Here's how the part is built. I have some questions about the finished solid (model axes, mm). A direction names the side the tool comes from. Coordinates: 2 decimals unless noted, no trailing zeros. Loops run counter-clockwise (first coordinate to the right, second up) from the corner with the lowest first, then second, coordinate; pieces in that order, holes last. Notation, with made-up numbers: M 45,88 L 69,88 A31 ccw 69,124 Z; hole C -24.5,-20 d11. An arc over 180 degrees is marked long. Use one line per item in the form item = value. Start each with the question number.
(1) On a 3-axis mill with a long thin cutter (end or side, diameter ignored), from which of +Z, -Z, +X, -X, +Y, -Y can I reach the whole of each face in a straight line? I mean faces 4 (the flat face through (-14.2, 4, 3)), 5 (the flat face through (-17, 0, 3)), 6 (the flat face through (0, 10, 0)), 7 (the flat face through (-11.5, -14, 0)). Say none if no direction works.
(2) Imagine slicing it at C-C, the plane y = -11.5. Please give me the cut outline in (x, z).
(3) Thinking about a two-plate mould opening in Y: for faces 1 (the flat face through (18.534, 13.728, 0.01)), 2 (the flat face through (-19, 1, 0)), 3 (the cylindrical face through (-13.706, -14.519, -0.01)), which applies, +Y half, -Y half, draft (parallel to the pull), parting line (faces both ways), or undercut?
(4) Imagine slicing it at A-A, the plane x = 14. Please give me the cut outline in (y, z).
(5) Imagine slicing it at B-B, the plane z = 2.7. Please give me the cut outline in (x, y).
(6) Will these pins go through, and if not, where does the flat tip stop? P1, Ø3.5, axis at x = 14.77, y = -15, coming from the +Z side; P2, Ø0.8, axis at y = -13.5, z = 0, coming from the -X side; P3, Ø0.8, axis at y = -13.5, z = 0, coming from the +X side.
(7) Imagine slicing it at D-D, the plane y = 15. Please give me the cut outline in (x, z) (3 decimals), and give its area (3 significant figures).
(8) Please list where these lines run through material, in increasing order: L1, parallel to Y at x = -14.5, z = 1.55; L2, parallel to Z at x = -7.5, y = 6.5; L3, parallel to Y at x = -4.5, z = -0.1.
```python
from build123d import *

# Parameters (mm, degrees)
F0_R     = 1.6
F1_DEPTH = 0.75
F2_W     = 5
F2_H     = 8
F3_DEPTH = 4
F4_W     = 7.2
F4_H     = 3.6
F5_DEPTH = 4.8


with BuildPart() as f1:
    # F0 (on Top) → F1 (new body, symmetric)
    with BuildSketch(Plane.XY):
        with BuildLine():
            Line((11, 10), (-11, 10))
            ThreePointArc((-11, 10), (-11.353553, 10.146447), (-11.5, 10.5))
            Line((-11.5, 10.5), (-11.5, 17.5))
            ThreePointArc((-11.5, 17.5), (-11.646447, 17.853553), (-12, 18))
            Line((-12, 18), (-17.558609, 18))
            ThreePointArc((-17.558609, 18), (-17.88951, 17.874839), (-18.054748, 17.562017))
            Line((-18.054748, 17.562017), (-19, 10))
            Line((-19, 10), (-19, 0))
            Line((-19, 0), (-19, -10))
            Line((-19, -10), (-18.054748, -17.562017))
            ThreePointArc((-18.054748, -17.562017), (-17.88951, -17.874839), (-17.558609, -18))
            Line((-17.558609, -18), (-12, -18))
            ThreePointArc((-12, -18), (-11.646447, -17.853553), (-11.5, -17.5))
            Line((-11.5, -17.5), (-11.5, -10.5))
            ThreePointArc((-11.5, -10.5), (-11.353553, -10.146447), (-11, -10))
            Line((-11, -10), (11, -10))
            ThreePointArc((11, -10), (11.353553, -10.146447), (11.5, -10.5))
            Line((11.5, -10.5), (11.5, -17.5))
            ThreePointArc((11.5, -17.5), (11.646447, -17.853553), (12, -18))
            Line((12, -18), (17.558609, -18))
            ThreePointArc((17.558609, -18), (17.88951, -17.874839), (18.054748, -17.562017))
            Line((18.054748, -17.562017), (19, -10))
            Line((19, -10), (19, 0))
            Line((19, 0), (19, 10))
            Line((19, 10), (18.054748, 17.562017))
            ThreePointArc((18.054748, 17.562017), (17.88951, 17.874839), (17.558609, 18))
            Line((17.558609, 18), (12, 18))
            ThreePointArc((12, 18), (11.646447, 17.853553), (11.5, 17.5))
            Line((11.5, 17.5), (11.5, 10.5))
            ThreePointArc((11.5, 10.5), (11.353553, 10.146447), (11, 10))
        make_face()
        with Locations((-15.232269, -15)):
            Circle(F0_R, mode=Mode.SUBTRACT)
        with Locations((14.767731, -15)):
            Circle(F0_R, mode=Mode.SUBTRACT)
        with Locations((-15.232269, 15)):
            Circle(F0_R, mode=Mode.SUBTRACT)
        with Locations((14.767731, 15)):
            Circle(F0_R, mode=Mode.SUBTRACT)
    extrude(amount=F1_DEPTH, both=True)

    # F2 (on face) → F3 (join)
    with BuildSketch(Plane.XY.offset(0.75)):
        with Locations((-16.5, 4)):
            Rectangle(F2_W, F2_H)
    extrude(amount=F3_DEPTH)

    # F4 (on face) → F5 (cut)
    with BuildSketch(Plane(origin=(-19, 0, 0), x_dir=(0, -1, 0), z_dir=(-1, 0, 0))):
        with Locations((-4, 2.75)):
            Rectangle(F4_W, F4_H)
    extrude(amount=-F5_DEPTH, mode=Mode.SUBTRACT)


solid = f1.part
```
Answer:
q1.face_4 = -X
q1.face_5 = +Z, +X, -X, -Y
q1.face_6 = +Z, -Z, +Y
q1.face_7 = +Z, -Z, -Y
q2.outline = M -18.81,-0.75 L -11.5,-0.75 L -11.5,0.75 L -18.81,0.75 Z; M 11.5,-0.75 L 18.81,-0.75 L 18.81,0.75 L 11.5,0.75 Z
q3.face_1 = +Y half
q3.face_2 = draft
q3.face_3 = undercut
q4.outline = M -18,-0.75 L -16.4,-0.75 L -16.4,0.75 L -18,0.75 Z; M -13.6,-0.75 L 13.6,-0.75 L 13.6,0.75 L -13.6,0.75 Z; M 16.4,-0.75 L 18,-0.75 L 18,0.75 L 16.4,0.75 Z
q5.outline = M -19,0 L -14,0 L -14,8 L -19,8 L -19,7.6 L -14.2,7.6 L -14.2,0.4 L -19,0.4 Z
q6.P1 = 0.75
q6.P2 = -18.61
q6.P3 = 18.61
q7.outline = M -18.375,-0.75 L -16.832,-0.75 L -16.832,0.75 L -18.375,0.75 Z; M -13.632,-0.75 L -11.5,-0.75 L -11.5,0.75 L -13.632,0.75 Z; M 11.5,-0.75 L 13.168,-0.75 L 13.168,0.75 L 11.5,0.75 Z; M 16.368,-0.75 L 18.375,-0.75 L 18.375,0.75 L 16.368,0.75 Z
q7.area = 11.0 mm²
q8.L1 = 0 to 0.4, 7.6 to 8
q8.L2 = -0.75 to 0.75
q8.L3 = -10 to 10
